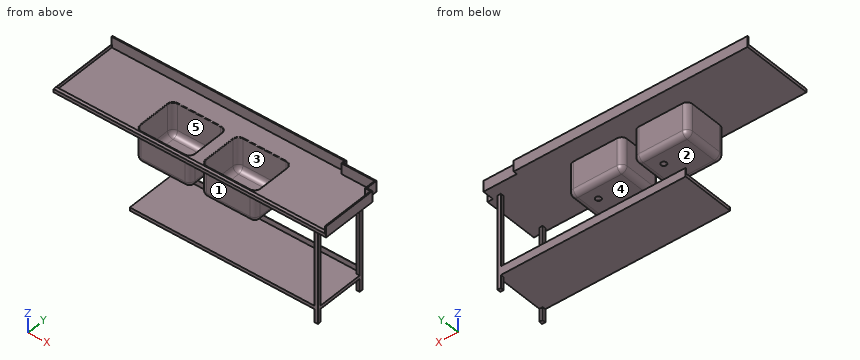
from build123d import *

# Parameters (mm, degrees)
F1_DEPTH     = 100
F3_DEPTH     = 98
F4_W         = 500
F4_H         = 400
F5_DEPTH     = 300
F6_W         = 2490
F6_H         = 30
F7_DEPTH     = 70
F8_T         = 2
F8_T3_DEPTH  = 104
F8_T5_DEPTH  = 34
F8_T7_DEPTH  = 32
F8_T9_DEPTH  = 102
F8_T11_DEPTH = 504
F8_T13_DEPTH = 404
F8_T15_DEPTH = 504
F9_R         = 50
F10_R        = 25
F11_DEPTH    = 2
F12_W        = 30
F12_H        = 30
F13_DEPTH    = 865
F14_R        = 6
F15_W        = 2
F15_H        = 28
F16_DEPTH    = 610
F18_DEPTH    = 1725


# Not quite as in the source:
# - a shell that OpenCascade refuses in one call is made with other operations: the cavity is built on its own and cut out
# - a feature names something its author has since deleted; it is built from what else it names


with BuildPart() as f1:
    # F0 (on Top) → F1 (new body)
    with BuildSketch(Plane.XY):
        Polygon((0, 650), (0, 0), (2500, 0), (2500, 510), (2450, 510), (2450, 615), (2145, 615), (2145, 650), align=None)
    extrude(amount=F1_DEPTH)

    # F2 (on face) → F3 (cut)
    with BuildSketch(Plane.XY.offset(100)):
        Polygon((0, 640), (0, 30), (2490, 30), (2490, 500), (2440, 500), (2440, 605), (2135, 605), (2135, 640), align=None)
    extrude(amount=-F3_DEPTH, mode=Mode.SUBTRACT)

    # F4 (on face) → F5 (join)
    with BuildSketch(Plane.XY.offset(2)):
        with Locations((950, 265)):
            Rectangle(F4_W, F4_H)
        with Locations((1550, 265)):
            Rectangle(F4_W, F4_H)
    extrude(amount=-F5_DEPTH)

    # F6 (on face) → F7 (cut)
    with BuildSketch(Plane.XY.offset(100)):
        with Locations((1245, 15)):
            Rectangle(F6_W, F6_H)
    extrude(amount=-F7_DEPTH, mode=Mode.SUBTRACT)

    # F8: shell of thickness 2, made by hand


with BuildPart() as f8_core1:
    # F8_t2: copy of F1
    add(f1.part)

    # the walls: a layer under each face that stays
    f8_faces = [f8_core1.faces().sort_by_distance(p)[0] for p in [
        (0, 21.6666666667, 23.3333333333),
        (1072.5, 650, 50),
        (2145, 632.5, 50),
        (2297.5, 615, 50),
        (2450, 562.5, 50),
        (2475, 510, 50),
        (2500, 255, 50),
        (97.65625, 641.975308642, 100),
        (2490, 250, 51),
        (2465, 500, 51),
        (2440, 552.5, 51),
        (2287.5, 605, 51),
        (2135, 622.5, 51),
        (1067.5, 640, 51),
        (1245, 30, 16),
        (1245, 15, 30),
        (416.6666666667, 0, 16.6666666667),
        (1250, 325, 0),
        (1800, 265, -149),
        (1550, 265, -298),
        (1550, 65, -149),
        (1300, 265, -149),
        (1550, 465, -149),
        (1200, 265, -149),
        (950, 265, -298),
        (950, 65, -149),
        (700, 265, -149),
        (950, 465, -149),
    ]]
    thicken(f8_faces, amount=-F8_T, mode=Mode.SUBTRACT)

    # F8_s4 → F8_t3 (cut)
    with BuildSketch(Plane.XY.offset(-2)):
        Polygon((2145.02, 615.02), (2143, 615), (2143, 613), (2145, 613), align=None)
        Polygon((2450.02, 510.02), (2448, 510), (2448, 508), (2450, 508), align=None)
    extrude(amount=F8_T3_DEPTH, mode=Mode.SUBTRACT)

    # F8_s6 → F8_t5 (cut)
    with BuildSketch(Plane.XZ.offset(-32)):
        Polygon((2489.98, 30.02), (2492, 30), (2492, 28), (2490, 28), align=None)
    extrude(amount=F8_T5_DEPTH, mode=Mode.SUBTRACT)

    # F8_s8 → F8_t7 (cut)
    with BuildSketch(Plane.XY):
        Polygon((2489.98, 30.02), (2492, 30), (2492, 28), (2490, 28), align=None)
    extrude(amount=F8_T7_DEPTH, mode=Mode.SUBTRACT)

    # F8_s10 → F8_t9 (cut)
    with BuildSketch(Plane.XY):
        Polygon((2489.98, 499.98), (2492, 500), (2492, 502), (2490, 502), align=None)
        Polygon((2439.98, 604.98), (2442, 605), (2442, 607), (2440, 607), align=None)
        Polygon((2134.98, 639.98), (2137, 640), (2137, 642), (2135, 642), align=None)
    extrude(amount=F8_T9_DEPTH, mode=Mode.SUBTRACT)

    # F8_s12 → F8_t11 (cut)
    with BuildSketch(Plane.YZ.offset(698)):
        Polygon((465.02, -0.02), (465, 2), (463, 2), (463, 0), align=None)
        Polygon((64.98, -0.02), (65, 2), (67, 2), (67, 0), align=None)
    extrude(amount=F8_T11_DEPTH, mode=Mode.SUBTRACT)

    # F8_s14 → F8_t13 (cut)
    with BuildSketch(Plane.XZ.offset(-467)):
        Polygon((699.98, -0.02), (700, 2), (702, 2), (702, 0), align=None)
        Polygon((1200.02, -0.02), (1200, 2), (1198, 2), (1198, 0), align=None)
        Polygon((1299.98, -0.02), (1300, 2), (1302, 2), (1302, 0), align=None)
        Polygon((1800.02, -0.02), (1800, 2), (1798, 2), (1798, 0), align=None)
    extrude(amount=F8_T13_DEPTH, mode=Mode.SUBTRACT)

    # F8_s16 → F8_t15 (cut)
    with BuildSketch(Plane.YZ.offset(1298)):
        Polygon((465.02, -0.02), (465, 2), (463, 2), (463, 0), align=None)
        Polygon((64.98, -0.02), (65, 2), (67, 2), (67, 0), align=None)
    extrude(amount=F8_T15_DEPTH, mode=Mode.SUBTRACT)


with BuildPart() as f1_1:
    add(f1.part)

    # what is left inside the walls is the cavity
    f8_cavity = [f8_core1.part.solids().sort_by_distance(p)[0] for p in [
        (1072.5, 647.98, 66),
        (950, 199, -295.98),
        (1550, 199, -295.98),
    ]]
    add(f8_cavity, mode=Mode.SUBTRACT)

    # F9
    f9_edges = [f1_1.edges().sort_by_distance(p)[0] for p in [
        (702, 463, -147),
        (1198, 463, -147),
        (950, 463, -296),
        (702, 67, -147),
        (1198, 67, -147),
        (1198, 265, -296),
        (950, 67, -296),
        (702, 265, -296),
        (1302, 265, -296),
        (1302, 463, -147),
        (1550, 463, -296),
        (1798, 463, -147),
        (1798, 265, -296),
        (1798, 67, -147),
        (1550, 67, -296),
        (1302, 67, -147),
        (700, 65, -149),
        (700, 265, -298),
        (950, 65, -298),
        (1300, 65, -149),
        (1300, 265, -298),
        (1550, 65, -298),
        (1200, 65, -149),
        (1200, 265, -298),
        (1800, 65, -149),
        (1800, 265, -298),
        (1800, 465, -149),
        (1550, 465, -298),
        (1300, 465, -149),
        (1200, 465, -149),
        (950, 465, -298),
        (700, 465, -149),
    ]]
    fillet(f9_edges, radius=F9_R)

    # F10 (on face) → F11 (cut, through all)
    with BuildSketch(Plane.XY.offset(-296)):
        with Locations((1048, 313)):
            Circle(F10_R)
        with Locations((1648, 313)):
            Circle(F10_R)
    extrude(amount=-F11_DEPTH, mode=Mode.SUBTRACT)

    # F12 (on face) → F13 (join)
    with BuildSketch(Plane(origin=(0, 0, 0), x_dir=(1, 0, 0), z_dir=(0, 0, -1))):
        with Locations((2385, -505)):
            Rectangle(F12_W, F12_H)
        with Locations((2385, -45)):
            Rectangle(F12_W, F12_H)
    extrude(amount=F13_DEPTH)

    # F14
    f14_edges = [f1_1.edges().sort_by_distance(p)[0] for p in [
        (950, 463, 2),
        (716.644661, 448.355339, 2),
        (1183.355339, 448.355339, 2),
        (702, 265, 2),
        (1198, 265, 2),
        (716.644661, 81.644661, 2),
        (1183.355339, 81.644661, 2),
        (950, 67, 2),
        (1550, 463, 2),
        (1316.644661, 448.355339, 2),
        (1783.355339, 448.355339, 2),
        (1302, 265, 2),
        (1798, 265, 2),
        (1316.644661, 81.644661, 2),
        (1783.355339, 81.644661, 2),
        (1550, 67, 2),
    ]]
    fillet(f14_edges, radius=F14_R)

    # F15 (on face) → F16 (join, through all)
    with BuildSketch(Plane(origin=(0, 30, 0), x_dir=(-1, 0, 0), z_dir=(0, 1, 0))):
        with Locations((-1, 16)):
            Rectangle(F15_W, F15_H)
    extrude(amount=F16_DEPTH)

    # F17 (on face) → F18 (join)
    with BuildSketch(Plane.YZ.offset(2400)):
        Polygon((30, -745), (520, -745), (520, -665), (518, -665), (518, -715), (30, -715), align=None)
    extrude(amount=-F18_DEPTH)


solid = f1_1.part
Source: CAD feature listing. Evaluate the final solid. Frame: model axes, mm. Face numbers are marked on the shaded views. A direction names the side the tool comes from. Coordinates: 2 decimals unless noted, no trailing zeros. Loops run counter-clockwise (first coordinate to the right, second up) from the corner with the lowest first, then second, coordinate; pieces in that order, holes last. Notation, with made-up numbers: (66.25, 7.25) - (92.25, 7.25) arc R33 ccw to (92.25, 41.25) - close; hole circle Ø7 at (89.5, -25). An arc over 180 degrees is marked (long way). Return JSON: item names as keys, results as strings.
Q1. Material intervals for line 1 along Y through (x, z) = (930, 29.5); line 2 along Z through (x, y) = (1276.5, 334); line 3 along Z through (x, y) = (1498, 359), sorted ascending.
Results:
{"line 1": "0 to 30, 640 to 642, 648 to 650", "line 2": "-745 to -715, 0 to 2", "line 3": "-745 to -715, -298 to -296"}
Q2. Section D-D, the plane y = 313. Give the number of separate pieces and of enclosed holes in the cut face, plus the area to 3 significant figures.
Results:
{"separate pieces": "4", "enclosed holes": "1", "area": "59,400 mm2"}
Q3. Section C-C, the plane x = 541. Return loops of the section in (y, z).
Results:
{"outline": "(0, 0) - (650, 0) - (650, 100) - (640, 100) - (640, 2) - (30, 2) - (30, 30) - (0, 30) - close; hole (2, 2) - (28, 2) - (28, 28) - (2, 28) - close; hole (642, 2) - (648, 2) - (648, 98) - (642, 98) - close"}
Q4. Mould query, pull axis Z, two halves, no side actions, for the marked faces 4 and 5. Classes: released by +Z, released by -Z, zero draft, split by the parting line, or undercut.
Results:
{"face 4": "undercut", "face 5": "zero draft"}
Q5. Access query for the marked faces 1, 2 and 3. Directions: +Z, -Z, +X, -X, +Y, -Y. A direction counts if a zero-diameter tool reaches every point of the face in a straight line with its end or side. Return the directions, or none.
Results:
{"face 1": "+X, -X, -Y", "face 2": "+X, -X, +Y, -Y", "face 3": "+Z"}
Q6. Contact query for flat-ended pins moving along their axis: P1, Ø3, axis at x = 808, y = 401.5, coming from the -Z side; P2, Ø1, axis at x = 1310.5, y = 518.5, coming from the +Z side; P3, Ø3, axis at y = 433.5, z = -28, coming from the +X side. Output: stop coordinate, or through.
Results:
{"P1": "z = -745", "P2": "z = 2", "P3": "x = 1797.02"}
Q7. Section A-A, the plane x = 1883. Return loops of the section in (y, z).
Results:
{"outline": "(0, 0) - (650, 0) - (650, 100) - (640, 100) - (640, 2) - (30, 2) - (30, 30) - (0, 30) - close; (30, -745) - (520, -745) - (520, -665) - (518, -665) - (518, -715) - (30, -715) - close; hole (2, 2) - (28, 2) - (28, 28) - (2, 28) - close; hole (642, 2) - (648, 2) - (648, 98) - (642, 98) - close"}
Q8. Section B-B, the plane z = -350.5. Return loops of the section in (x, y).
Results:
{"outline": "(2370, 30) - (2400, 30) - (2400, 60) - (2370, 60) - close; (2370, 490) - (2400, 490) - (2400, 520) - (2370, 520) - close"}
